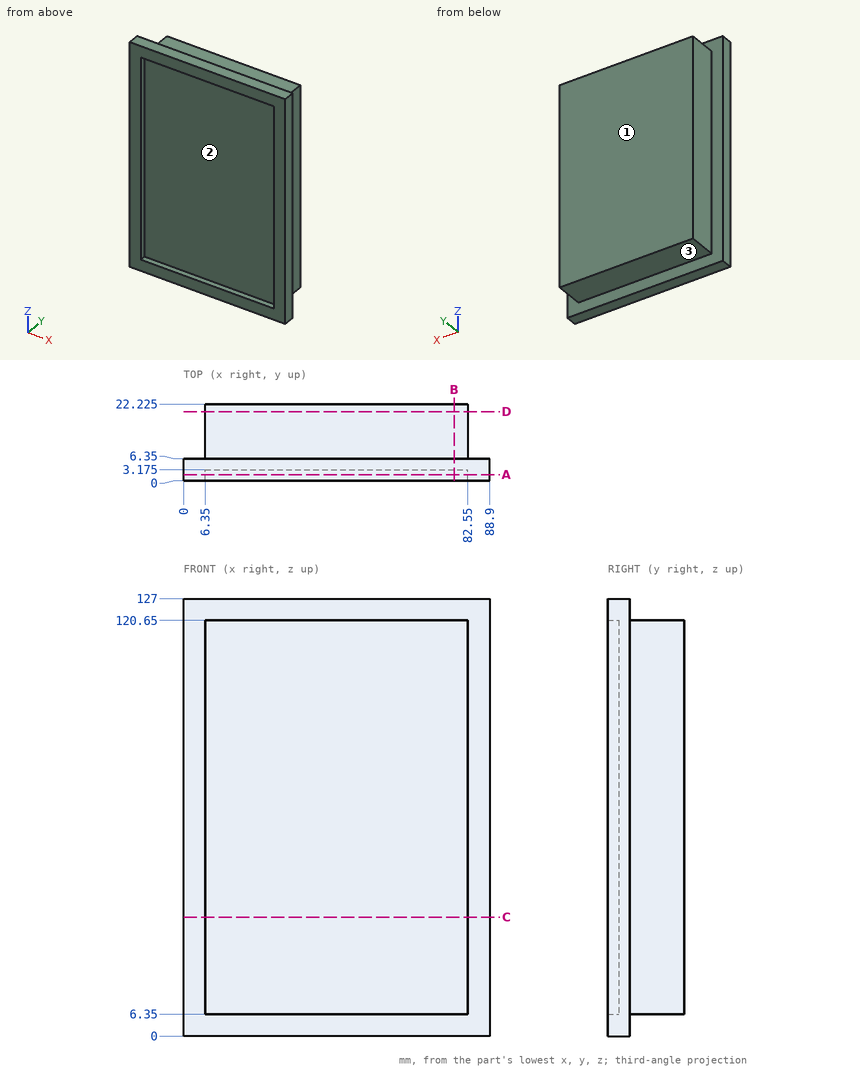
Here's the drawing with two shaded views (mm, measured from the low corner). I have some questions. Round coordinates to 2 decimals unless told otherwise and drop trailing zeros. Order: outer loops, then holes, each group sorted by start corner. A loop starts at its lowest first (then second) coordinate and runs counter-clockwise, first axis right, second up. Notation, with made-up numbers: (58, 69.5) -> (98, 69.5) arc R34 cw to (98, 105.5) -> close; hole circle Ø8 at (29, 47). An arc over 180 degrees is marked (long way). Write each question's results on one line, items separated by ' | '. Start each with the question number.
Item 1: If we section it at C-C, the plane z = 34.5: Write out the boundary of the cut face in (x, y) (3 decimals), then the cut area to 3 significant figures.
Item 2: If we section it at B-B, the plane x = 78.5: Write out the boundary of the cut face in (y, z) (3 decimals).
Item 3: If we section it at D-D, the plane y = 20: Write out the boundary of the cut face in (x, z).
Item 4: Thinking about a two-plate mould opening in Z: for the marked faces 1, 2 and 3, which applies, +Z half, -Z half, draft (parallel to the pull), parting line (faces both ways), or undercut?
Item 5: Please list where these lines run through material, in increasing order: L1, parallel to Z at x = 80, y = 11.75; L2, parallel to Y at x = 50, z = 104.5 (3 decimals); L3, parallel to Y at x = 74.5, z = 121.
Item 6: If we section it at A-A, the plane y = 1.75: Write out the boundary of the cut face in (x, z), then the cut area to 3 significant figures.
Item 7: Will these pins go through, and if not, where does the flat tip stop? pin 1 (4 mm diameter, centred on x = 65, y = 19, fed in from -Z); pin 2 (5 mm diameter, centred on y = 9, z = 40, fed in from +X); pin 3 (5 mm diameter, centred on y = 15, z = 64.5, fed in from -X).
Results:
1) outline: (0, 0) -> (6.35, 0) -> (6.35, 3.175) -> (82.55, 3.175) -> (82.55, 0) -> (88.9, 0) -> (88.9, 6.35) -> (82.55, 6.35) -> (82.55, 22.225) -> (6.35, 22.225) -> (6.35, 6.35) -> (0, 6.35) -> close | area: 1,530 mm2
2) outline: (0, 0) -> (6.35, 0) -> (6.35, 6.35) -> (22.225, 6.35) -> (22.225, 120.65) -> (6.35, 120.65) -> (6.35, 127) -> (0, 127) -> (0, 120.65) -> (3.175, 120.65) -> (3.175, 6.35) -> (0, 6.35) -> close
3) outline: (6.35, 6.35) -> (82.55, 6.35) -> (82.55, 120.65) -> (6.35, 120.65) -> close
4) face 1: draft | face 2: undercut | face 3: -Z half
5) L1: z = 6.35 to 120.65 | L2: y = 3.175 to 22.225 | L3: y = 0 to 6.35
6) outline: (0, 0) -> (88.9, 0) -> (88.9, 127) -> (0, 127) -> close; hole (6.35, 6.35) -> (82.55, 6.35) -> (82.55, 120.65) -> (6.35, 120.65) -> close | area: 2,580 mm2
7) pin 1: stops at z = 6.35 | pin 2: stops at x = 82.55 | pin 3: stops at x = 6.35
